Design review of the part built by this model. Coordinates are the model's own, in mm. A direction names the side the tool comes from. Coordinates: 2 decimals unless noted, no trailing zeros. Write each loop counter-clockwise with the first axis right and the second up, starting at its lowest first coordinate (ties: lowest second). Pieces come first, ordered by that corner, then holes. Notation, with made-up numbers: (9, -19) -> (33, -19) arc R17 cw to (33, -13) -> close; hole circle Ø8 at (32, 40.25). An arc over 180 degrees is marked (long way). One line per question, with ' | ' between items. Start each with the question number.
Q1. Add section A-A on y = -1. State the section outline as (x, z) points.
Q2. Wall thickness on probe 1 along Z at (x, y) = (0, 16); probe 2 along X at (y, z) = (6.5, 26.5); probe 3 along Y at (x, z) = (-24.5, 16): over which ranges is each line inside the solid? List them lowest first.
Q3. Add section B-B on x = 0. State the section outline as (y, z) points, and give its area (3 significant figures).
Q4. Add section D-D on z = 11. State the section outline as (x, y) points.
Q5. Add section C-C on x = -13.5. State the section outline as (y, z) points.
Q6. For P1, Ø5, axis at y = 13.5, z = 15, coming from the +X side; P2, Ø1.5, axis at x = 29, z = 14.5, coming from the +Y side; P3, Ø2, axis at x = 33.5, y = -17.5, coming from the +Z side; P4, Ø4, axis at x = 0, z = 28, coming from the +Y side, all flat-tipped, find the tip position at first contact; note any pin that passes through.
Q7. Draft analysis for pull direction Y (two halves, no side actions). For faces 5 (the flat face through (-1, -20, 6)), 6 (the cylindrical face through (-44, -28, 3)), 7 (the flat face through (0, 14.5, 19)), state which applies: pulls with the +Y half, pulls with the -Y half, needs draft (parallel to the pull), parting line crosses it, or undercut.
Q8. For faces 1 (the flat face through (-17.52, -14.75, 28.14)), 2 (the flat face through (-32.5, 0, 22)), 3 (the cylindrical face through (-31.64, -17.1, 22.22)), 4 (the cylindrical face through (31.6, 17.14, 22.22)), list the 3-axis set-ups (+Z, -Z, +X, -X, +Y, -Y) from which the entire face can be reached by the end or side of a thin tool; tool diameter is ignored.
from build123d import *

# Parameters (mm, degrees)
F0_W      = 90
F0_H      = 60
F1_DEPTH  = 6
F2_W      = 65
F2_H      = 36
F3_DEPTH  = 32
F4_W      = 58
F4_H      = 29
F5_DEPTH  = 38
F7_DEPTH  = 3.5
F8_R      = 2.5
F9_DEPTH  = 3.5
F11_DEPTH = 12
F12_R     = 5.5
F12_R_2   = 4
F13_DEPTH = 2
F14_DEPTH = 25
F15_R     = 5
F16_R     = 3


with BuildPart() as f1:
    # F0 (on Top) → F1 (new body)
    with BuildSketch(Plane.XY):
        Rectangle(F0_W, F0_H)
    extrude(amount=F1_DEPTH)

    # F2 (on face) → F3 (join)
    with BuildSketch(Plane.XY.offset(6)):
        Rectangle(F2_W, F2_H)
    extrude(amount=F3_DEPTH)

    # F4 (on face) → F5 (cut, through all)
    with BuildSketch(Plane.XY.offset(38)):
        Rectangle(F4_W, F4_H)
    extrude(amount=-F5_DEPTH, mode=Mode.SUBTRACT)

    # F6 (on face) → F7 (cut, through all)
    with BuildSketch(Plane.XZ.offset(18)):
        Polygon((19, 38), (-19, 38), (-16, 18), (0, 18), (16, 18), align=None)
    extrude(amount=-F7_DEPTH, mode=Mode.SUBTRACT)

    # F8 (on face) → F9 (cut, through all)
    with BuildSketch(Plane.XZ.offset(-14.5)):
        with Locations((0, 28)):
            Circle(F8_R)
    extrude(amount=-F9_DEPTH, mode=Mode.SUBTRACT)

    # F10 (on face) → F11 (cut, through all)
    with BuildSketch(Plane(origin=(0, 30, 0), x_dir=(-1, 0, 0), z_dir=(0, 1, 0))):
        with BuildLine():
            Line((10.9752045511, 6), (-10.9752045511, 6))
            ThreePointArc((-10.9752045511, 6), (0, 0.532957507), (10.9752045511, 6))
        make_face()
    extrude(amount=-F11_DEPTH, mode=Mode.SUBTRACT)

    # F12 (on face) → F13 (join)
    with BuildSketch(Plane(origin=(0, 18, 0), x_dir=(-1, 0, 0), z_dir=(0, 1, 0))):
        with Locations((0, 11)):
            Circle(F12_R)
        with Locations((0, 11)):
            Circle(F12_R_2, mode=Mode.SUBTRACT)
    extrude(amount=F13_DEPTH)

    # F14 (cut): a face of the model
    f14_faces = [f1.faces().sort_by_distance(p)[0] for p in [
        (0, 18, 11),
    ]]
    extrude(f14_faces, amount=-F14_DEPTH, mode=Mode.SUBTRACT)

    # F15
    f15_edges = [f1.edges().sort_by_distance(p)[0] for p in [
        (45, -30, 3),
        (45, 30, 3),
        (-45, -30, 3),
        (-45, 30, 3),
    ]]
    fillet(f15_edges, radius=F15_R)

    # F16
    f16_edges = [f1.edges().sort_by_distance(p)[0] for p in [
        (-32.5, 18, 22),
        (-32.5, -18, 22),
        (32.5, 18, 22),
        (32.5, -18, 22),
        (-17.5, -18, 28),
        (17.5, -18, 28),
        (0, -18, 18),
    ]]
    fillet(f16_edges, radius=F16_R)


solid = f1.part
Output values:
1) outline: (-45, 0) -> (-29, 0) -> (-29, 38) -> (-32.5, 38) -> (-32.5, 6) -> (-45, 6) -> close; (29, 0) -> (45, 0) -> (45, 6) -> (32.5, 6) -> (32.5, 38) -> (29, 38) -> close
2) probe 1: z = 0 to 7, 15 to 25.5, 30.5 to 38 | probe 2: x = -32.5 to -29, 29 to 32.5 | probe 3: y = -18 to -14.5, 14.5 to 18
3) outline: (-30, 0) -> (-14.5, 0) -> (-14.5, 18) -> (-15, 18) arc R3 ccw to (-18, 15) -> (-18, 6) -> (-30, 6) -> close; (14.5, 0) -> (30, 0) -> (30, 0.53) -> (18, 0.53) -> (18, 5.5) -> (20, 5.5) -> (20, 7) -> (14.5, 7) -> close; (14.5, 15) -> (20, 15) -> (20, 16.5) -> (18, 16.5) -> (18, 25.5) -> (14.5, 25.5) -> close; (14.5, 30.5) -> (18, 30.5) -> (18, 38) -> (14.5, 38) -> close | area: 233 mm2
4) outline: (-32.5, -15) arc R3 ccw to (-29.5, -18) -> (29.5, -18) arc R3 ccw to (32.5, -15) -> (32.5, 15) arc R3 ccw to (29.5, 18) -> (5.5, 18) -> (5.5, 20) -> (4, 20) -> (4, 14.5) -> (29, 14.5) -> (29, -14.5) -> (-29, -14.5) -> (-29, 14.5) -> (-4, 14.5) -> (-4, 20) -> (-5.5, 20) -> (-5.5, 18) -> (-29.5, 18) arc R3 ccw to (-32.5, 15) -> close
5) outline: (-30, 0) -> (-14.5, 0) -> (-14.5, 18) -> (-15, 18) arc R3 ccw to (-18, 15) -> (-18, 6) -> (-30, 6) -> close; (14.5, 0) -> (30, 0) -> (30, 6) -> (18, 6) -> (18, 38) -> (14.5, 38) -> close
6) P1: stops at x = 32.5 | P2: stops at y = 18 | P3: stops at z = 6 | P4: passes through
7) face 5: needs draft | face 6: pulls with the -Y half | face 7: undercut
8) face 1: +Z, -Y | face 2: +Z, -X, +Y, -Y | face 3: +Z, -X, -Y | face 4: +Z, +X, +Y
